Part model, mm, in its own coordinate system. Face numbers are marked on the shaded views. A direction names the side the tool comes from. Coordinates: 2 decimals unless noted, no trailing zeros. Loops run counter-clockwise (first coordinate to the right, second up) from the corner with the lowest first, then second, coordinate; pieces in that order, holes last. Notation, with made-up numbers: (42, -34) - (62, -34) arc R33 ccw to (62, 1) - close; hole circle Ø1 at (-3, 70.5). An arc over 180 degrees is marked (long way). Answer as CSV lines item,"result".
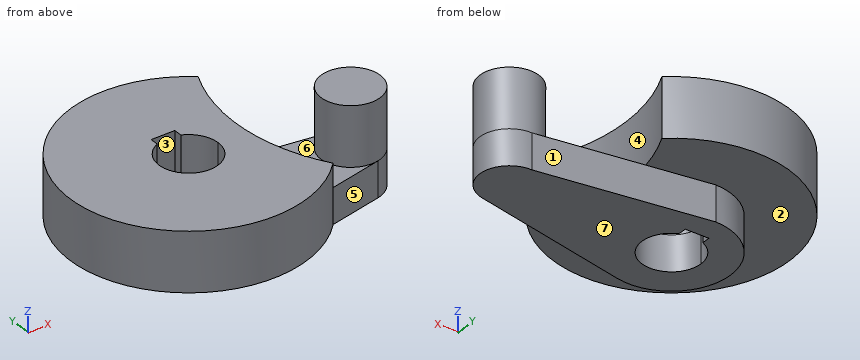
from build123d import *
from build123d.topology import SkipClean

# Parameters (mm, degrees)
SKETCH_1_R          = 10
SKETCH_1_R_2        = 2.5
EXTRUDE_1_DEPTH     = 5
SKETCH_2_R          = 15
CUT_EXTRUDE_1_DEPTH = 5
EXTRUDE_START       = 3
SKETCH_3_R          = 2.5
EXTRUDE_2_DEPTH     = 3
SKETCH_4_R          = 2.5
EXTRUDE_3_DEPTH     = 5
SKETCH_5_W          = 2
SKETCH_5_H          = 1
CUT_EXTRUDE_2_DEPTH = 21.990484753


with BuildPart() as part:
    # 草图1 → 凸台-拉伸1 (new body)
    with BuildSketch(Plane.XY):
        Circle(SKETCH_1_R)
        Circle(SKETCH_1_R_2, mode=Mode.SUBTRACT)
    extrude(amount=EXTRUDE_1_DEPTH)

    # 草图2 → 切除-拉伸1 (cut)
    with BuildSketch(Plane(origin=(0, 0, 0), x_dir=(-1, 0, 0), z_dir=(0, 0, -1))):
        with Locations((-19.955808724, 1.328795767)):
            Circle(SKETCH_2_R)
    extrude(amount=-CUT_EXTRUDE_1_DEPTH, mode=Mode.SUBTRACT)

    # 草图3 → 凸台-拉伸2 (add)
    with SkipClean():  # the faces are left unmerged after this step: merging them gives an invalid solid
        with BuildSketch(Plane(origin=(0, 0, 0), x_dir=(-1, 0, 0), z_dir=(0, 0, -1)).offset(EXTRUDE_START)):
            with BuildLine():
                Line((-14.033505879, 3.051346054), (0.163638991, 4.997321511))
                ThreePointArc((0.163638991, 4.997321511), (4.961120501, -0.622320962), (-1.075733127, -4.882908789))
                Line((-1.075733127, -4.882908789), (-14.669175898, -1.888194504))
                ThreePointArc((-14.669175898, -1.888194504), (-16.610861535, 0.872353736), (-14.033505879, 3.051346054))
            make_face()
            Circle(SKETCH_3_R, mode=Mode.SUBTRACT)
        extrude(amount=-EXTRUDE_2_DEPTH)

    # 草图4 → 凸台-拉伸3 (add)
    with SkipClean():  # the faces are left unmerged after this step: merging them gives an invalid solid
        with BuildSketch(Plane.XY):
            with Locations((14.131309334, 0.55325989)):
                Circle(SKETCH_4_R)
        extrude(amount=EXTRUDE_3_DEPTH)

    # 草图5 → 切除-拉伸2 (cut, through all)
    with SkipClean():  # the faces are left unmerged after this step: merging them gives an invalid solid
        with BuildSketch(Plane.XY.offset(5)):
            with Locations((0, 2.5)):
                Rectangle(SKETCH_5_W, SKETCH_5_H)
        extrude(amount=-CUT_EXTRUDE_2_DEPTH, mode=Mode.SUBTRACT)
    add(part.part.scale(1), mode=Mode.REPLACE)  # the faces are merged on a copy


solid = part.part
Q1. Two-plate mould, pull along X, no slides. Class the marked faces 1, 2, 3 and 4: released by +X, released by -X, zero draft, split by the parting line, or undercut.
Results:
face 1,"released by +X"
face 2,"zero draft"
face 3,"undercut"
face 4,"undercut"
Q2. Saw through at B-B (z = 3.5). Give the cut face in (x, y).
Results:
outline,"(6.38, 7.7) arc R10 ccw (long way) to (7.34, -6.79) arc R15 cw to start; circle Ø5 at (14.13, 0.55); hole (-1, 2.29) arc R2.5 ccw (long way) to (1, 2.29) - (1, 3) - (-1, 3) - close"
Q3. Saw through at D-D (y = -3.5). Give the cut face in (x, z).
Results:
outline,"(-9.37, 0) - (-3.57, 0) - (-3.57, -3) - (7.35, -3) - (7.35, 0) - (5.75, 0) - (5.75, 5) - (-9.37, 5) - close"
Q4. Saw through at C-C (y = -1.25). Give the cut face in (x, z).
Results:
outline,"(-9.92, 0) - (-4.84, 0) - (-4.84, -3) - (-2.17, -3) - (-2.17, 5) - (-9.92, 5) - close; (2.17, -3) - (15.86, -3) - (15.86, 5) - (12.4, 5) - (12.4, 0) - (5.18, 0) - (5.18, 5) - (2.17, 5) - close"
Q5. Saw through at A-A (z = -0.5). Give the cut face in (x, y), then the cut area to 3 significant figures.
Results:
outline,"(-0.16, 5) arc R5 ccw (long way) to (1.08, -4.88) - (14.67, -1.89) arc R2.5 ccw to (14.03, 3.05) - close; hole (-1, 2.29) arc R2.5 ccw (long way) to (1, 2.29) - (1, 3) - (-1, 3) - close"
area,"135 mm^2"
Q6. Which spindle directions (+Z, -Z, +X, -X, +Y, -Y) get a long thin tool onto all of the face, cutting with end or side? Do the marked faces 5, 6 and 7. Say none if no direction does.
Results:
face 5,"-Z, +X, -Y"
face 6,"+Z"
face 7,"-Z, +X, -X, +Y, -Y"
Q7. Wall check: L1, parallel to X at y = 0.75, z = 1.75; L2, parallel to Y at x = 0, z = 3.2; L3, parallel to X at y = 0, z = 1.15. Give the ranges that are in metal, low to high.
Results:
L1,"x = -9.97 to -2.38, 2.38 to 4.97, 11.64 to 16.62"
L2,"y = -10 to -2.5, 3 to 10"
L3,"x = -10 to -2.5, 2.5 to 5.01, 11.69 to 16.57"
Q8. Flat gauge pins, fed straight in: pin 1 (1 mm diameter, centred on y = 4, z = 3.5, fed in from +X); pin 2 (1.5 mm diameter, centred on x = -7, y = 0.5, fed in from -Z); pin 3 (2 mm diameter, centred on x = -4, z = 1, fed in from -Y); pin 4 (4.5 mm diameter, centred on x = 0, y = 0, fed in from -Z). Where does each tip first touch, or does it go through?
Results:
pin 1,"stops at x = 5.29"
pin 2,"stops at z = 0"
pin 3,"stops at y = -9.54"
pin 4,"passes through"
